Part model, mm, in its own coordinate system. Face numbers are marked on the shaded views. A direction names the side the tool comes from. Round coordinates to 2 decimals unless told otherwise and drop trailing zeros. Order: outer loops, then holes, each group sorted by start corner. A loop starts at its lowest first (then second) coordinate and runs counter-clockwise, first axis right, second up. Notation, with made-up numbers: (18.25, -27) -> (28.25, -27) arc R30 ccw to (28.25, 6) -> close; hole circle Ø2 at (-14.75, -32.75). An arc over 180 degrees is marked (long way). Use CSV: the item, a comma, the result in double quotes.
Autodesk Fusion 360 part; units mm, degrees
sketch "Sketch1" plane through (0, 0, 0) normal (0, 0, 1) x (1, 0, 0)
  line L0 (0, 0) -> (105, 0)
  line L1 (105, 0) -> (105, 55)
  line L2 (105, 55) -> (0, 55)
  line L3 (0, 55) -> (0, 0)
  dimension "d1" = 105
  dimension "d2" = 55
extrude "Extrude1" add sketch "Sketch1" along normal blind 18
sketch "Sketch2" plane through (0, 0, 18) normal (0, 0, 1) x (-1, 0, 0)
  line L0 (0, -55) -> (0, 0)
  line L1 (0, 0) -> (-105, 0)
  line L2 (-105, 0) -> (-105, -55)
  line L3 (-105, -55) -> (0, -55)
  line L4 (0, -55) -> (-105, 0) construction
  line L5 (-105, -55) -> (0, 0) construction
  line L6 (-52.5, -27.5) -> (-52.5, -42) construction
  line L7 (-52.5, -42) -> (-92, -42)
  line L8 (-92, -42) -> (-92, -13)
  line L9 (-92, -13) -> (-13, -13)
  line L10 (-13, -13) -> (-13, -42)
  line L11 (-13, -42) -> (-52.5, -42)
  dimension "d5" = 29
  dimension "d6" = 79
  dimension "d7" = 14.5
  dimension "d8" = 39.5
extrude "Extrude2" cut sketch "Sketch2" against normal blind 5 contours L7 L8 L9 L10 L11
fillet "Fillet1" radius 6 4 edges at (13, 42, 15.5) (92, 42, 15.5) (92, 13, 15.5) (13, 13, 15.5)
sketch "Sketch3" plane through (0, 0, 13) normal (0, 0, 1) x (-1, 0, 0)
  arc A0 (-13, -19) -> (-19, -13) centre (-19, -19) ccw
  line L0 (-19, -13) -> (-86, -13)
  arc A1 (-86, -13) -> (-92, -19) centre (-86, -19) ccw
  line L1 (-92, -19) -> (-92, -36)
  arc A2 (-92, -36) -> (-86, -42) centre (-86, -36) ccw
  line L2 (-86, -42) -> (-19, -42)
  arc A3 (-19, -42) -> (-13, -36) centre (-19, -36) ccw
  line L3 (-13, -36) -> (-13, -19)
  line L4 (0, -55) -> (-105, 0) construction
  line L5 (-105, 0) -> (-105, -55) construction
  line L6 (-105, -55) -> (0, 0) construction
  line L7 (-52.5, -27.5) -> (-33, -27.5) construction
  line L8 (-52.5, -27.5) -> (-72, -27.5) construction
  dimension "d13" = 19.5
  dimension "d14" = 19.5
hole "Hole1" at (0, 0, 0) at (72, 27.5, 13) at (33, 27.5, 13) direction (0, 0, -1) diameter 10 depth 10 tip angle 180
equation "d7 = ( 29 / 2 ) * 1 mm"
equation "d8 = ( 79 / 2 ) * 1 mm"
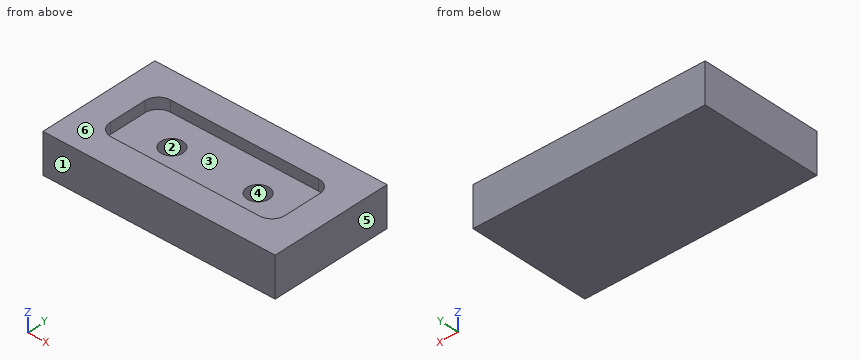
(1) Cut at C-C, the plane x = 33. Give the cut face in (y, z).
Reply:
outline,"(0, 0) -> (55, 0) -> (55, 18) -> (42, 18) -> (42, 13) -> (32.5, 13) -> (32.5, 3) -> (22.5, 3) -> (22.5, 13) -> (13, 13) -> (13, 18) -> (0, 18) -> close"
(2) Cut at B-B, the plane z = 9. Give the cut face in (x, y), then the cut area to 3 significant figures.
Reply:
outline,"(0, 0) -> (105, 0) -> (105, 55) -> (0, 55) -> close; hole circle Ø10 at (33, 27.5); hole circle Ø10 at (72, 27.5)"
area,"5,620 mm2"
(3) Cut at D-D, the plane z = 15.75. Give the cut face in (x, y), then the cut area to 3 significant figures.
Reply:
outline,"(0, 0) -> (105, 0) -> (105, 55) -> (0, 55) -> close; hole (13, 19) arc R6 ccw to (19, 13) -> (86, 13) arc R6 ccw to (92, 19) -> (92, 36) arc R6 ccw to (86, 42) -> (19, 42) arc R6 ccw to (13, 36) -> close"
area,"3,510 mm2"
(4) Which spindle directions (+Z, -Z, +X, -X, +Y, -Y) get a long thin tool onto all of the face, cutting with end or side? Do the marked faces 1 and 2. Say none if no direction does.
Reply:
face 1,"+Z, -Z, +X, -X, -Y"
face 2,"+Z"
(5) Cut at A-A, the plane y = 27.5. Give the cut face in (x, z).
Reply:
outline,"(0, 0) -> (105, 0) -> (105, 18) -> (92, 18) -> (92, 13) -> (77, 13) -> (77, 3) -> (67, 3) -> (67, 13) -> (38, 13) -> (38, 3) -> (28, 3) -> (28, 13) -> (13, 13) -> (13, 18) -> (0, 18) -> close"
(6) Pull direction X, two halves, no side cores. Call the marked faces 3, 4, 5 and 6: released by +X, released by -X, zero draft, split by the parting line, or undercut.
Reply:
face 3,"undercut"
face 4,"undercut"
face 5,"released by +X"
face 6,"zero draft"
(7) Drop flat-ended pins along their axis: P1, Ø9, axis at x = 72, y = 27.5, coming from the +Z side; P2, Ø8.5, axis at x = 49, y = 22, coming from the +Z side. Give the stop position or say it passes through.
Reply:
P1,"z = 3"
P2,"z = 13"
(8) Probe probe 1 along X at (y, z) = (27.5, 10.25); probe 2 along Y at (x, z) = (72, 10); probe 3 along Z at (x, y) = (25, 18). List the from-to ranges inside material, lowest first. Write a range as [from, to].
Reply:
probe 1,"[0, 28], [38, 67], [77, 105]"
probe 2,"[0, 22.5], [32.5, 55]"
probe 3,"[0, 13]"
